Check sheet for the modelled part. Datum: model origin and axes. Units: mm. Face numbers are marked on the shaded views. A direction names the side the tool comes from. Round coordinates to 2 decimals unless told otherwise and drop trailing zeros. Loops run counter-clockwise (first coordinate to the right, second up) from the corner with the lowest first, then second, coordinate; pieces in that order, holes last. Notation, with made-up numbers: (82, 0.5) - (120, 0.5) arc R31 ccw to (120, 25.5) - close; hole circle Ø1 at (53.25, 17.25). An arc over 180 degrees is marked (long way). Answer in a Markdown table with one row per item. Add a question column.
(1) Cross-section at D-D on x = -24.5. Enter the section's corners in (y, z), then the cut area to 3 significant figures.
(2) Cross-section at B-B on x = -3. Enter the section's corners in (y, z), then the cut area to 3 significant figures.
(3) Gauge pin test, flat ends, axial feed: pin 1 (1.8 mm diameter, centred on x = -29.5, z = -13.5, fed in from +Y); pin 2 (1.1 mm diameter, centred on y = 0.5, z = -3, fed in from -X); pin 3 (1.1 mm diameter, centred on x = -18, y = 0.5, fed in from +Z). Record the tip position at first contact, or that the pin passes through.
(4) Thickness scan on line 1 along Z through (x, y) = (-3, 0.3); line 2 along Y through (x, z) = (-13, -14); line 3 along X through (y, z) = (2, -11.75). Record the ranges inside material, lowest first.
(5) Cross-section at A-A on z = -13.5. Enter the section's corners in (x, y).
(6) Cross-section at C-C on y = 11.5. Enter the section's corners in (x, z).
(7) Access from +Z, -Z, +X, -X, +Y, -Y to the whole of each face (thin tool, end or side, straight path). Record for the marked faces 1 and 2.
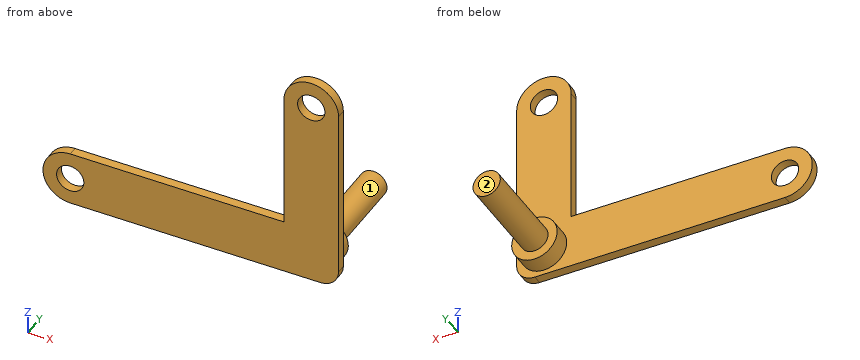
Autodesk Inventor part; units mm, degrees
ref_plane "YZ Plane" through (0, 0, 0) normal (1, 0, 0) x (0, 1, 0)
ref_plane "XZ Plane" through (0, 0, 0) normal (0, 1, 0) x (-1, 0, 0)
ref_plane "XY Plane" through (0, 0, 0) normal (0, 0, 1) x (1, 0, 0)
sketch "Sketch1" plane through (0, 0, 0) normal (0, 1, 0) x (-1, 0, 0)
  circle A0 centre (3, -13.5) radius 1.5
  circle A1 centre (29.5, -13.5) radius 1.5
  circle A2 centre (29.5, -13.5) radius 3
  circle A3 centre (3, 4.5) radius 1.5
  circle A4 centre (3, 4.5) radius 3
  line L0 (29.5, -16.5) -> (0, -16.5)
  line L1 (0, -16.5) -> (0, 4.5)
  line L2 (29.5, -10.5) -> (6, -10.5)
  line L3 (6, -10.5) -> (6, 4.5)
  point P0 (0, 0)
  dimension "d24" = 3
  dimension "d57" = 3
  dimension "d58" = 6
  dimension "d59" = 3
  dimension "d60" = 6
ref_plane "Work Plane1" through (0, 1, 0) normal (0, 1, 0) x (1, 0, 0)
sketch "Sketch2" plane through (0, 1, 0) normal (0, 1, 0) x (1, 0, 0)
  line L0 (0, -4.5) -> (0, 14.5)
  circle A0 centre (-3, 13.5) radius 1.5
  circle A1 centre (-3, 13.5) radius 1.5
  circle A2 centre (-3, 13.5) radius 2.5
  point P0 (0, 0)
  point P1 (-6, 10.5)
  dimension "d36" = 5
extrude "Extrusion5" add sketch "Sketch2" along normal blind 2
extrude "Extrusion6" add sketch "Sketch2" along normal blind 12 and the other way blind 1 contours A0
thread "Thread2"
extrude "Extrusion8" add sketch "Sketch1" along normal blind 1
fillet "Fillet3" radius 2 1 edges at (0, 0.5, -16.5)
properties part number "linkToActuator2"
Answers:
| question | item | result |
|---|---|---|
| 1 | outline | (0, -16.5) - (1, -16.5) - (1, -10.5) - (0, -10.5) - close |
| 1 | area | 6.00 mm^2 |
| 2 | outline | (0, -16.5) - (1, -16.5) - (1, -16) - (3, -16) - (3, -15) - (13, -15) - (13, -12) - (3, -12) - (3, -11) - (1, -11) - (1, 3) - (0, 3) - close; (0, 6) - (1, 6) - (1, 7.5) - (0, 7.5) - close |
| 2 | area | 61.0 mm^2 |
| 3 | pin 1 | passes through |
| 3 | pin 2 | stops at x = -6 |
| 3 | pin 3 | stops at z = -10.5 |
| 4 | line 1 | z = -16.5 to 3, 6 to 7.5 |
| 4 | line 2 | y = 0 to 1 |
| 4 | line 3 | x = -4.79 to -1.21 |
| 5 | outline | (-32.5, 0) - (-31, 0) - (-31, 1) - (-32.5, 1) - close; (-28, 0) - (0, 0) - (0, 1) - (-0.5, 1) - (-0.5, 3) - (-1.5, 3) - (-1.5, 13) - (-4.5, 13) - (-4.5, 3) - (-5.5, 3) - (-5.5, 1) - (-28, 1) - close |
| 6 | outline | circle Ø3 at (-3, -13.5) |
| 7 | face 1 | +Y |
| 7 | face 2 | +Z, -Z, +X, -X, +Y |
